Autodesk Inventor part; units mm, degrees
ref_plane "bspg_1_XY" through (30, -4.6, 0) normal (1, 0, 0) x (0, 0, -1)
ref_plane "bspg_1_YZ" through (30, -4.6, 0) normal (0, 0, -1) x (0, 1, 0)
ref_plane "bspg_1_ZX" through (30, -4.6, 0) normal (0, 1, 0) x (1, 0, 0)
sketch "Sketch_1" plane through (0, 0, 0) normal (1, 0, 0) x (0, 1, 0)
  line L0 (-7, 7.5) -> (-7, 6.3)
  line L1 (-7, 6.3) -> (-2.5, 6.3)
  arc A0 (-1.2, 5) -> (-2.5, 6.3) centre (-2.5, 5) ccw
  line L2 (-1.2, 5) -> (-1.2, -5)
  arc A1 (-2.5, -6.3) -> (-1.2, -5) centre (-2.5, -5) ccw
  line L3 (-2.5, -6.3) -> (-7, -6.3)
  line L4 (-7, -6.3) -> (-7, -7.5)
  line L5 (-7, -7.5) -> (-2.79, -7.5)
  arc A2 (-2.79, -7.5) -> (0, -4.71) centre (-2.79, -4.71) ccw
  line L6 (0, -4.71) -> (0, 4.71)
  arc A3 (0, 4.71) -> (-2.79, 7.5) centre (-2.79, 4.71) ccw
  line L7 (-2.79, 7.5) -> (-7, 7.5)
extrude "Extrusion1" add sketch "Sketch_1" along normal blind 60
sketch "Sketch_2" plane through (0.02, 0, 0) normal (1, 0, 0) x (0, 0, -1)
  line L0 (-6.3, -7) -> (-5.95, -7)
  line L1 (-5.95, -7) -> (-5.6669, -3.9266)
  arc A0 (-4.8703, -3.2) -> (-5.6669, -3.9266) centre (-4.8703, -4) ccw
  line L2 (-4.8703, -3.2) -> (4.8703, -3.2)
  arc A1 (5.6669, -3.9266) -> (4.8703, -3.2) centre (4.8703, -4) ccw
  line L3 (5.6669, -3.9266) -> (5.95, -7)
  line L4 (5.95, -7) -> (6.3, -7)
  line L5 (6.3, -7) -> (6.3, -2.5)
  arc A2 (6.3, -2.5) -> (5, -1.2) centre (5, -2.5) ccw
  line L6 (5, -1.2) -> (-5, -1.2)
  arc A3 (-5, -1.2) -> (-6.3, -2.5) centre (-5, -2.5) ccw
  line L7 (-6.3, -2.5) -> (-6.3, -7)
extrude "Extrusion2" add sketch "Sketch_2" along normal blind 1.4
sketch "Sketch_3" plane through (59.98, 0, 0) normal (1, 0, 0) x (0, 0, -1)
  line L0 (-6.3, -7) -> (-5.95, -7)
  line L1 (-5.95, -7) -> (-5.6669, -3.9266)
  arc A0 (-4.8703, -3.2) -> (-5.6669, -3.9266) centre (-4.8703, -4) ccw
  line L2 (-4.8703, -3.2) -> (4.8703, -3.2)
  arc A1 (5.6669, -3.9266) -> (4.8703, -3.2) centre (4.8703, -4) ccw
  line L3 (5.6669, -3.9266) -> (5.95, -7)
  line L4 (5.95, -7) -> (6.3, -7)
  line L5 (6.3, -7) -> (6.3, -2.5)
  arc A2 (6.3, -2.5) -> (5, -1.2) centre (5, -2.5) ccw
  line L6 (5, -1.2) -> (-5, -1.2)
  arc A3 (-5, -1.2) -> (-6.3, -2.5) centre (-5, -2.5) ccw
  line L7 (-6.3, -2.5) -> (-6.3, -7)
extrude "Extrusion3" add sketch "Sketch_3" against normal blind 1.4
sketch "Sketch_4" plane through (10, 0, 0) normal (1, 0, 0) x (0, 0, -1)
  line L0 (0, -1.2) -> (0, 0)
  line L1 (0, 0) -> (1.5, 0)
  line L2 (1.5, 0) -> (1.2295, -0.2705)
  line L3 (1.2295, -0.2705) -> (1.2295, -0.9295)
  line L4 (1.2295, -0.9295) -> (1.5, -1.2)
  line L5 (1.5, -1.2) -> (0, -1.2)
  line L6 (0, -1.2) -> (0, 0)
revolve "Revolution1" cut sketch "Sketch_4" angle 360 about axis through (10, -1.2, 0) along (0, -1, 0)
thread "Thread1"
sketch "Sketch_5" plane through (50, 0, 0) normal (1, 0, 0) x (0, 0, -1)
  line L0 (0, -1.2) -> (0, 0)
  line L1 (0, 0) -> (1.5, 0)
  line L2 (1.5, 0) -> (1.2295, -0.2705)
  line L3 (1.2295, -0.2705) -> (1.2295, -0.9295)
  line L4 (1.2295, -0.9295) -> (1.5, -1.2)
  line L5 (1.5, -1.2) -> (0, -1.2)
  line L6 (0, -1.2) -> (0, 0)
revolve "Revolution2" cut sketch "Sketch_5" angle 360 about axis through (50, -1.2, 0) along (0, -1, 0)
thread "Thread2"
sketch "Sketch6" plane through (1.42, -1.2, -5) normal (0, -1, 0) x (1, 0, 0)
  point P0 (36.13, 5)
hole "Hole1" at (37.55, -1.2, 0) direction (0, 1, 0) diameter 1.8 depth 1.2
sketch "Sketch7" plane through (1.42, -1.2, -5) normal (0, -1, 0) x (1, 0, 0)
  point P0 (21.03, 5)
hole "Hole2" at (22.45, -1.2, 0) direction (0, 1, 0) diameter 1.8 depth 1.2
sketch "Sketch_9" plane through (30, 0, 0) normal (1, 0, 0) x (0, 0, -1)
  arc A0 (-5.75, -3.5) -> (-5.75, -5.7) centre (-5.75, -4.6) ccw
  line L0 (-5.75, -5.7) -> (-5.75, -3.5)
extrude "Extrusion4" cut sketch "Sketch_9" along normal mid plane 36
sketch "Sketch_10" plane through (30, 0, 0) normal (1, 0, 0) x (0, 0, -1)
  line L0 (5.75, -3.5) -> (5.75, -5.7)
  arc A0 (5.75, -5.7) -> (5.75, -3.5) centre (5.75, -4.6) ccw
extrude "Extrusion5" cut sketch "Sketch_10" along normal mid plane 36
ref_plane "bspg_1_XY" through (30, -4.6, 0) normal (1, 0, 0) x (0, 0, -1)
ref_plane "bspg_1_YZ" through (30, -4.6, 0) normal (0, 0, -1) x (0, 1, 0)
ref_plane "bspg_1_ZX" through (30, -4.6, 0) normal (0, 1, 0) x (1, 0, 0)
ref_plane "bspg_1r_XY" through (30, -3.5, 0) normal (1, 0, 0) x (0, 0, -1)
ref_plane "bspg_1r_YZ" through (30, -3.5, 0) normal (0, 0, -1) x (0, 1, 0)
ref_plane "bspg_1r_ZX" through (30, -3.5, 0) normal (0, 1, 0) x (1, 0, 0)
ref_plane "bspg_d_XY" through (0, 0, 0) normal (0, 1, 0) x (1, 0, 0)
ref_plane "bspg_d_YZ" through (0, 0, 0) normal (1, 0, 0) x (0, 0, -1)
ref_plane "bspg_d_ZX" through (0, 0, 0) normal (0, 0, -1) x (0, 1, 0)
properties part number "BSPG1560 Table"
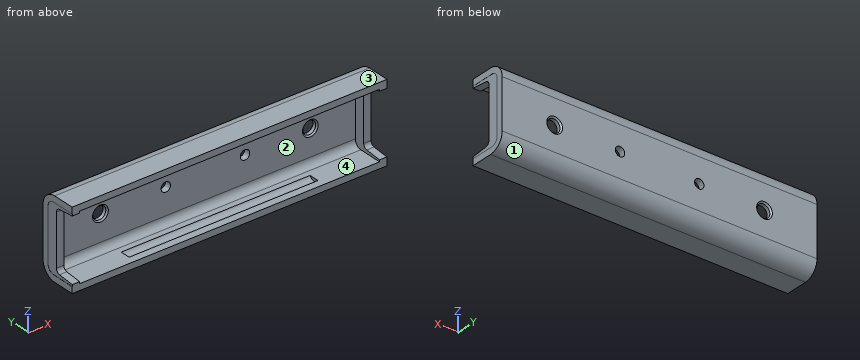
Here's how the part is built. I have some questions about the finished solid (model axes, mm). Face numbers are marked on the shaded views. A direction names the side the tool comes from. Coordinates: 2 decimals unless noted, no trailing zeros. Write each loop counter-clockwise with the first axis right and the second up, starting at its lowest first coordinate (ties: lowest second). Pieces come first, ordered by that corner, then holes.
Item 1: Will these pins go through, and if not, where does the flat tip stop? pin 1 (2 mm diameter, centred on x = 22.45, z = 0, fed in from -Y); pin 2 (2 mm diameter, centred on x = 12.5, y = -0.5, fed in from -Z); pin 3 (4 mm diameter, centred on x = 26, z = -2, fed in from +Y); pin 4 (1.1 mm diameter, centred on x = 59, z = -2, fed in from -Y).
Item 2: I want a section at A-A on x = 22.45. Write out the boundary of the cut face in (y, z).
Item 3: I want a section at D-D on x = 10. Write out the boundary of the cut face in (y, z).
Item 4: If I drill on line 1 (X direction, y = -0.5, z = 0); line 2 (X direction, y = -6.5, z = -6.25); line 3 (Z direction, x = 30, y = -4.5), over which ranges is the centre line in solid material (lowest first)?
Item 5: On a 3-axis mill with a long thin cutter (end or side, diameter ignored), from which of +Z, -Z, +X, -X, +Y, -Y can I reach the whole of each face in a straight line? I mean the marked faces 1 and 2. Say none if no direction works.
Item 6: If we mould it in two halves opening along X, with no side actions, what happens to the marked faces 3 and 4? For each: +X half, -X half, draft (parallel to the pull), parting line (faces both ways), or undercut.
Findings below:
1. pin 1: stops at y = -1.2
1. pin 2: stops at z = -7.18
1. pin 3: stops at y = 0
1. pin 4: stops at y = -3.2
2. outline: (-7, -7.5) - (-2.79, -7.5) arc R2.79 ccw to (0, -4.71) - (0, -0.9) - (-1.2, -0.9) - (-1.2, -5) arc R1.3 cw to (-2.5, -6.3) - (-3.65, -6.3) arc R1.1 cw to (-5.55, -6.3) - (-7, -6.3) - close; (-7, 6.3) - (-5.55, 6.3) arc R1.1 cw to (-3.65, 6.3) - (-2.5, 6.3) arc R1.3 cw to (-1.2, 5) - (-1.2, 0.9) - (0, 0.9) - (0, 4.71) arc R2.79 ccw to (-2.79, 7.5) - (-7, 7.5) - close
3. outline: (-7, -7.5) - (-2.79, -7.5) arc R2.79 ccw to (0, -4.71) - (0, -1.5) - (-0.27, -1.23) - (-0.93, -1.23) - (-1.2, -1.5) - (-1.2, -5) arc R1.3 cw to (-2.5, -6.3) - (-7, -6.3) - close; (-7, 6.3) - (-2.5, 6.3) arc R1.3 cw to (-1.2, 5) - (-1.2, 1.5) - (-0.93, 1.23) - (-0.27, 1.23) - (0, 1.5) - (0, 4.71) arc R2.79 ccw to (-2.79, 7.5) - (-7, 7.5) - close
4. line 1: x = 0 to 8.77, 11.23 to 21.55, 23.35 to 36.65, 38.45 to 48.77, 51.23 to 60
4. line 2: x = 0.02 to 1.42, 58.58 to 59.98
4. line 3: z = -7.5 to -6.85, 6.85 to 7.5
5. face 1: -Z, +X, -X, +Y
5. face 2: -Y
6. face 3: draft
6. face 4: undercut
